Input: part model. Units: mm. Frame: model coordinates. Face numbers are marked on the shaded views. Coordinates: 2 decimals unless noted, no trailing zeros. Loops run counter-clockwise (first coordinate to the right, second up) from the corner with the lowest first, then second, coordinate; pieces in that order, holes last.
(1) Section D-D, the plane y = 42.5. Return loops of the section in (x, z).
(2) Section C-C, the plane y = 6. Give the number of separate pieces and of enclosed holes in the cut face, then the cut area to 3 significant figures.
(3) Contact query for flat-ended pins moving along their axis: P1, Ø1.7, axis at x = -51, z = 8.5, coming from the -Y side; P2, Ø8, axis at x = -46.5, z = -51.5, coming from the +Y side; P3, Ø6.5, axis at x = 0, z = 67.5, coming from the +Y side. Output: stop coordinate, or through.
(4) Mould query, pull axis X, two halves, no side actions, for the marked faces 1, 2 and 3. Classes: released by +X, released by -X, zero draft, split by the parting line, or undercut.
(5) Line query: L1, parallel to Y at x = 52.5, z = 67.25; L2, parallel to Y at x = -51.5, z = -38; L3, parallel to X at y = 38, z = 69. Output: solid intervals per line, ascending.
(6) Section A-A, the plane x = 31.5. Return loops of the section in (y, z).
(7) Section B-B, the plane z = -4. Return loops of the section in (x, y).
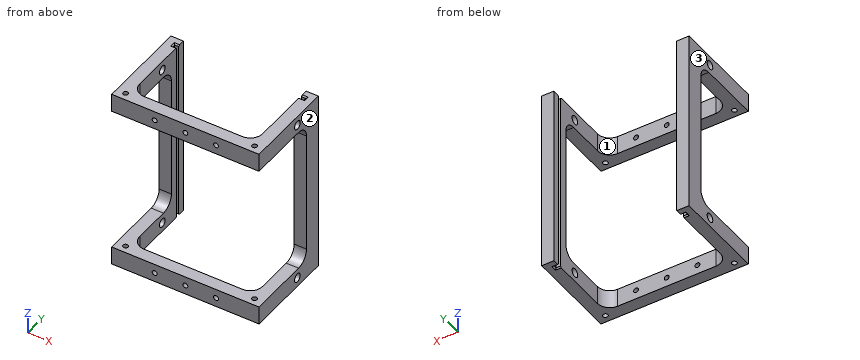
```python
from build123d import *

# Parameters (mm, degrees)
SKETCH1_W           = 120
SKETCH1_H           = 150
BOSS_EXTRUDE1_DEPTH = 75
SKETCH3_W           = 107
SKETCH3_H           = 2.5
CUT_EXTRUDE2_DEPTH  = 179.115131306
SKETCH2_W           = 100
SKETCH2_H           = 150
CUT_EXTRUDE1_DEPTH  = 65
FILLET1_R           = 10
SKETCH4_R           = 2
CUT_EXTRUDE3_DEPTH  = 116.974135047
SKETCH5_R           = 2
CUT_EXTRUDE4_DEPTH  = 179.115131306
SKETCH6_R           = 3.55
CUT_EXTRUDE5_DEPTH  = 161.15617378
CHAMFER1_SIZE       = 1
SKETCH7_W           = 120
SKETCH7_H           = 60
CUT_EXTRUDE6_DEPTH  = 161.15617378
FILLET2_R           = 10


with BuildPart() as part:
    # Sketch1 → Boss-Extrude1 (new body)
    with BuildSketch(Plane(origin=(0, 0, 0), x_dir=(1, 0, 0), z_dir=(0, 1, 0))):
        Rectangle(SKETCH1_W, SKETCH1_H)
    extrude(amount=BOSS_EXTRUDE1_DEPTH)

    # Sketch3 → Cut-Extrude2 (cut, through all)
    with BuildSketch(Plane.XY.offset(75)):
        with Locations((0.15445013, 68)):
            Rectangle(SKETCH3_W, SKETCH3_H)
    extrude(amount=-CUT_EXTRUDE2_DEPTH, mode=Mode.SUBTRACT)

    # Sketch2 → Cut-Extrude1 (cut)
    with BuildSketch(Plane(origin=(0, 75, 0), x_dir=(1, 0, 0), z_dir=(0, 1, 0))):
        Rectangle(SKETCH2_W, SKETCH2_H)
    extrude(amount=-CUT_EXTRUDE1_DEPTH, mode=Mode.SUBTRACT)

    # Fillet1
    fillet1_edges = [part.edges().sort_by_distance(p)[0] for p in [
        (50, 10, 0),
        (-50, 10, 0),
    ]]
    fillet(fillet1_edges, radius=FILLET1_R)

    # Sketch4 → Cut-Extrude3 (cut, through all)
    with BuildSketch(Plane(origin=(0, 10, 0), x_dir=(1, 0, 0), z_dir=(0, 1, 0))):
        with Locations(Location((0, 67.5, 0), (0, 0, 270))):
            Circle(SKETCH4_R)
        with Locations(Location((25, 67.5, 0), (0, 0, 270))):
            Circle(SKETCH4_R)
        with Locations(Location((-25, 67.5, 0), (0, 0, 270))):
            Circle(SKETCH4_R)
        with Locations(Location((-25, -67.5, 0), (0, 0, 90))):
            Circle(SKETCH4_R)
        with Locations(Location((25, -67.5, 0), (0, 0, 90))):
            Circle(SKETCH4_R)
        with Locations(Location((0, -67.5, 0), (0, 0, 90))):
            Circle(SKETCH4_R)
    extrude(amount=-CUT_EXTRUDE3_DEPTH, mode=Mode.SUBTRACT)

    # Sketch5 → Cut-Extrude4 (cut, through all)
    with BuildSketch(Plane.XY.offset(75)):
        with Locations((-52.5, 6)):
            Circle(SKETCH5_R)
        with Locations((52.5, 6)):
            Circle(SKETCH5_R)
    extrude(amount=-CUT_EXTRUDE4_DEPTH, mode=Mode.SUBTRACT)

    # Sketch6 → Cut-Extrude5 (cut, through all)
    with BuildSketch(Plane(origin=(60, 0, 0), x_dir=(0, 0, -1), z_dir=(1, 0, 0))):
        with Locations((67.5, 48.5)):
            Circle(SKETCH6_R)
        with Locations((-67.5, 48.5)):
            Circle(SKETCH6_R)
    extrude(amount=-CUT_EXTRUDE5_DEPTH, mode=Mode.SUBTRACT)

    # Chamfer1
    chamfer1_edges = [part.edges().sort_by_distance(p)[0] for p in [
        (53.65445013, 68, -75),
        (-51.672774935, 66.75, -75),
        (-53.34554987, 68, -75),
        (51.827225065, 69.25, -75),
        (53.65445013, 68, 75),
        (51.827225065, 69.25, 75),
        (-53.34554987, 68, 75),
        (-51.672774935, 66.75, 75),
        (-51.672774935, 69.25, 75),
        (-51.672774935, 69.25, -75),
        (51.827225065, 66.75, 75),
        (51.827225065, 66.75, -75),
    ]]
    chamfer(chamfer1_edges, length=CHAMFER1_SIZE)

    # Sketch7 → Cut-Extrude6 (cut, through all)
    with BuildSketch(Plane(origin=(60, 0, 0), x_dir=(0, 0, -1), z_dir=(1, 0, 0))):
        with Locations((0, 30)):
            Rectangle(SKETCH7_W, SKETCH7_H)
    extrude(amount=-CUT_EXTRUDE6_DEPTH, mode=Mode.SUBTRACT)

    # Fillet2
    fillet2_edges = [part.edges().sort_by_distance(p)[0] for p in [
        (55, 60, 60),
        (-55, 60, 60),
        (-55, 60, -60),
        (55, 60, -60),
    ]]
    fillet(fillet2_edges, radius=FILLET2_R)


solid = part.part
```
Report:
1. outline: (-60, -75) - (-50, -75) - (-50, -60) - (-60, -60) - close; (-60, 60) - (-50, 60) - (-50, 75) - (-60, 75) - close; (50, -75) - (60, -75) - (60, -60) - (50, -60) - close; (50, 60) - (60, 60) - (60, 75) - (50, 75) - close
2. separate pieces: 6
2. enclosed holes: 6
2. area: 3,280 mm2
3. P1: stops at y = 60
3. P2: stops at y = 75
3. P3: stops at y = 10
4. face 1: undercut
4. face 2: released by +X
4. face 3: released by -X
5. L1: y = 0 to 4, 8 to 44.96, 52.04 to 66.75, 69.25 to 75
5. L2: y = 60 to 66.75, 69.25 to 75
5. L3: x = -60 to -50, 50 to 60
6. outline: (0, -75) - (10, -75) - (10, -60) - (0, -60) - close; (0, 60) - (10, 60) - (10, 75) - (0, 75) - close
7. outline: (-60, 60) - (-50, 60) - (-50, 66.75) - (-53.35, 66.75) - (-53.35, 69.25) - (-50, 69.25) - (-50, 75) - (-60, 75) - close; (50, 60) - (60, 60) - (60, 75) - (50, 75) - (50, 69.25) - (53.65, 69.25) - (53.65, 66.75) - (50, 66.75) - close
